from build123d import *

# Parameters (mm, degrees)
F0_W          = 140
F0_H          = 45
F1_DEPTH      = 20
F2_W          = 100
F2_H          = 27
F3_DEPTH      = 25
F4_R          = 2.65
F5_DEPTH      = 45.001
F6_R          = 4.5
F7_DEPTH      = 25
F8_T1_DEPTH   = 80
F9_R          = 5
F10_T1_DEPTH  = 116
F10_T3_DEPTH  = 90
F10_T5_DEPTH  = 37
F10_T7_DEPTH  = 48
F10_T10_ANGLE = 90
F10_T12_ANGLE = 90
F10_T14_ANGLE = 89.9999999987
F10_T16_ANGLE = 89.9999999987
F10_T18_ANGLE = 90
F10_T20_ANGLE = 90
F10_T22_ANGLE = 89.9999999987
F10_T24_ANGLE = 89.9999999987


# Not quite as in the source:
# - a fillet or chamfer that OpenCascade refuses, or shapes differently, is made with other operations: its cross-section is extruded or revolved along the edge and cut away or added


with BuildPart() as f1:
    # F0 (on Top) → F1 (new body)
    with BuildSketch(Plane.XY):
        Rectangle(F0_W, F0_H)
    extrude(amount=F1_DEPTH)

    # F2 (on face) → F3 (cut)
    with BuildSketch(Plane.XY.offset(20)):
        with Locations((0, -9)):
            Rectangle(F2_W, F2_H)
    extrude(amount=-F3_DEPTH, mode=Mode.SUBTRACT)

    # F4 (on face) → F5 (cut, through all)
    with BuildSketch(Plane(origin=(0, 22.5, 0), x_dir=(-1, 0, 0), z_dir=(0, 1, 0))):
        with Locations((60, 10)):
            Circle(F4_R)
        with Locations((-60, 10)):
            Circle(F4_R)
    extrude(amount=-F5_DEPTH, mode=Mode.SUBTRACT)

    # F6 (on face) → F7 (cut)
    with BuildSketch(Plane(origin=(0, 22.5, 0), x_dir=(-1, 0, 0), z_dir=(0, 1, 0))):
        with Locations((60, 10)):
            Circle(F6_R)
        with Locations((-60, 10)):
            Circle(F6_R)
    extrude(amount=-F7_DEPTH, mode=Mode.SUBTRACT)

    # F8: fillet of radius 12 on 2 edges, made by hand

    # F8_s2 → F8_t1 (cut)
    with BuildSketch(Plane.XY.offset(-30)):
        with BuildLine():
            ThreePointArc((-58, 22.5), (-66.4852813742, 18.9852813742), (-70, 10.5))
            Line((-70, 10.5), (-70, 22.5))
            Line((-70, 22.5), (-58, 22.5))
        make_face()
        with BuildLine():
            ThreePointArc((58, 22.5), (66.4852813742, 18.9852813742), (70, 10.5))
            Line((70, 10.5), (70, 22.5))
            Line((70, 22.5), (58, 22.5))
        make_face()
    extrude(amount=F8_T1_DEPTH, mode=Mode.SUBTRACT)

    # F9
    f9_edges = [f1.edges().sort_by_distance(p)[0] for p in [
        (-50, 4.5, 10),
        (50, 4.5, 10),
    ]]
    fillet(f9_edges, radius=F9_R)

    # F10: fillet of radius 6 on 20 edges, made by hand

    # F10_s2 → F10_t1 (cut)
    with BuildSketch(Plane.YZ.offset(-58)):
        with BuildLine():
            ThreePointArc((22.5, 14), (20.7426406871, 18.2426406871), (16.5, 20))
            Line((16.5, 20), (22.5, 20))
            Line((22.5, 20), (22.5, 14))
        make_face()
        with BuildLine():
            ThreePointArc((16.5, 0), (20.7426406871, 1.7573593129), (22.5, 6))
            Line((22.5, 6), (22.5, 0))
            Line((22.5, 0), (16.5, 0))
        make_face()
    extrude(amount=F10_T1_DEPTH, mode=Mode.SUBTRACT)

    # F10_s4 → F10_t3 (cut)
    with BuildSketch(Plane.YZ.offset(-45)):
        with BuildLine():
            ThreePointArc((4.5, 14), (6.2573593129, 18.2426406871), (10.5, 20))
            Line((10.5, 20), (4.5, 20))
            Line((4.5, 20), (4.5, 14))
        make_face()
        with BuildLine():
            ThreePointArc((10.5, 0), (6.2573593129, 1.7573593129), (4.5, 6))
            Line((4.5, 6), (4.5, 0))
            Line((4.5, 0), (10.5, 0))
        make_face()
    extrude(amount=F10_T3_DEPTH, mode=Mode.SUBTRACT)

    # F10_s6 → F10_t5 (cut)
    with BuildSketch(Plane.XZ.offset(0.5)):
        with BuildLine():
            ThreePointArc((56, 0), (51.7573593129, 1.7573593129), (50, 6))
            Line((50, 6), (50, 0))
            Line((50, 0), (56, 0))
        make_face()
        with BuildLine():
            ThreePointArc((-56, 0), (-51.7573593129, 1.7573593129), (-50, 6))
            Line((-50, 6), (-50, 0))
            Line((-50, 0), (-56, 0))
        make_face()
        with BuildLine():
            ThreePointArc((50, 14), (51.7573593129, 18.2426406871), (56, 20))
            Line((56, 20), (50, 20))
            Line((50, 20), (50, 14))
        make_face()
        with BuildLine():
            ThreePointArc((-50, 14), (-51.7573593129, 18.2426406871), (-56, 20))
            Line((-56, 20), (-50, 20))
            Line((-50, 20), (-50, 14))
        make_face()
    extrude(amount=F10_T5_DEPTH, mode=Mode.SUBTRACT)

    # F10_s8 → F10_t7 (cut)
    with BuildSketch(Plane.XZ.offset(-10.5)):
        with BuildLine():
            ThreePointArc((64, 0), (68.2426406871, 1.7573593129), (70, 6))
            Line((70, 6), (70, 0))
            Line((70, 0), (64, 0))
        make_face()
        with BuildLine():
            ThreePointArc((-64, 0), (-68.2426406871, 1.7573593129), (-70, 6))
            Line((-70, 6), (-70, 0))
            Line((-70, 0), (-64, 0))
        make_face()
        with BuildLine():
            ThreePointArc((70, 14), (68.2426406871, 18.2426406871), (64, 20))
            Line((64, 20), (70, 20))
            Line((70, 20), (70, 14))
        make_face()
        with BuildLine():
            ThreePointArc((-70, 14), (-68.2426406871, 18.2426406871), (-64, 20))
            Line((-64, 20), (-70, 20))
            Line((-70, 20), (-70, 14))
        make_face()
    extrude(amount=F10_T7_DEPTH, mode=Mode.SUBTRACT)

    # F10_s9 → F10_t10 (revolve, cut)
    with BuildSketch(Plane.XZ.offset(0.5)):
        with BuildLine():
            ThreePointArc((56, 0), (51.7573593129, 1.7573593129), (50, 6))
            Line((50, 6), (50, 0))
            Line((50, 0), (56, 0))
        make_face()
    revolve(axis=Axis((45, -0.5, 0), (0, 0, 1)), revolution_arc=F10_T10_ANGLE, mode=Mode.SUBTRACT)

    # F10_s11 → F10_t12 (revolve, cut)
    with BuildSketch(Plane.YZ.offset(-45)):
        with BuildLine():
            ThreePointArc((10.5, 0), (6.2573593129, 1.7573593129), (4.5, 6))
            Line((4.5, 6), (4.5, 0))
            Line((4.5, 0), (10.5, 0))
        make_face()
    revolve(axis=Axis((-45, -0.5, 0), (0, 0, 1)), revolution_arc=F10_T12_ANGLE, mode=Mode.SUBTRACT)

    # F10_s13 → F10_t14 (revolve, cut)
    with BuildSketch(Plane.YZ.offset(57.9999999999)):
        with BuildLine():
            ThreePointArc((16.5, 0), (20.7426406871, 1.7573593129), (22.5, 6))
            Line((22.5, 6), (22.5, 0))
            Line((22.5, 0), (16.5, 0))
        make_face()
    revolve(axis=Axis((57.9999999999, 10.4999999999, 0), (0, 0, -1)), revolution_arc=F10_T14_ANGLE, mode=Mode.SUBTRACT)

    # F10_s15 → F10_t16 (revolve, cut)
    with BuildSketch(Plane.XZ.offset(-10.4999999999)):
        with BuildLine():
            ThreePointArc((-64, 0), (-68.2426406871, 1.7573593129), (-70, 6))
            Line((-70, 6), (-70, 0))
            Line((-70, 0), (-64, 0))
        make_face()
    revolve(axis=Axis((-57.9999999999, 10.4999999999, 0), (0, 0, -1)), revolution_arc=F10_T16_ANGLE, mode=Mode.SUBTRACT)

    # F10_s17 → F10_t18 (revolve, cut)
    with BuildSketch(Plane.XZ.offset(0.5)):
        with BuildLine():
            ThreePointArc((50, 14), (51.7573593129, 18.2426406871), (56, 20))
            Line((56, 20), (50, 20))
            Line((50, 20), (50, 14))
        make_face()
    revolve(axis=Axis((45, -0.5, 20), (0, 0, 1)), revolution_arc=F10_T18_ANGLE, mode=Mode.SUBTRACT)

    # F10_s19 → F10_t20 (revolve, cut)
    with BuildSketch(Plane.YZ.offset(-45)):
        with BuildLine():
            ThreePointArc((4.5, 14), (6.2573593129, 18.2426406871), (10.5, 20))
            Line((10.5, 20), (4.5, 20))
            Line((4.5, 20), (4.5, 14))
        make_face()
    revolve(axis=Axis((-45, -0.5, 20), (0, 0, 1)), revolution_arc=F10_T20_ANGLE, mode=Mode.SUBTRACT)

    # F10_s21 → F10_t22 (revolve, cut)
    with BuildSketch(Plane.YZ.offset(57.9999999999)):
        with BuildLine():
            ThreePointArc((22.5, 14), (20.7426406871, 18.2426406871), (16.5, 20))
            Line((16.5, 20), (22.5, 20))
            Line((22.5, 20), (22.5, 14))
        make_face()
    revolve(axis=Axis((57.9999999999, 10.4999999999, 20), (0, 0, -1)), revolution_arc=F10_T22_ANGLE, mode=Mode.SUBTRACT)

    # F10_s23 → F10_t24 (revolve, cut)
    with BuildSketch(Plane.XZ.offset(-10.4999999999)):
        with BuildLine():
            ThreePointArc((-70, 14), (-68.2426406871, 18.2426406871), (-64, 20))
            Line((-64, 20), (-70, 20))
            Line((-70, 20), (-70, 14))
        make_face()
    revolve(axis=Axis((-57.9999999999, 10.4999999999, 20), (0, 0, -1)), revolution_arc=F10_T24_ANGLE, mode=Mode.SUBTRACT)


solid = f1.part
Can you work these out from the model? Positions are in its coordinate system, mm. A direction names the side the tool comes from. Give positions to 0.01 mm unless a question says otherwise; leave off trailing zeros. Order: outer loops, then holes, each group sorted by start corner. A loop starts at its lowest first (then second) coordinate and runs counter-clockwise, first axis right, second up. Notation, with made-up numbers: M -33,-5.75 L 3,-5.75 A16 cw 3,14.25 Z; hole C 20,-7 d10. An arc over 180 degrees is marked long. Use one line per item in the form item = value.
Item 1: If I drill on line 1 along X through (y, z) = (8.75, 10); line 2 along X through (y, z) = (-19, 9.75); line 3 along Z through (x, y) = (-60, -9), over which ranges is the centre line in solid material (lowest first)? Write a range as [from, to].
Values follow:
line_1 = [-70, -64.5], [-55.5, 55.5], [64.5, 70]
line_2 = [-70, -62.64], [-57.36, -50], [50, 57.36], [62.64, 70]
line_3 = [0, 7.35], [12.65, 20]
Item 2: If we section it at D-D, the plane y = 8.5: Count the separate pieces of the cut face and the enclosed holes in it, and give its area (3 significant figures).
Values follow:
separate_pieces = 1
enclosed_holes = 2
area = 2,580 mm^2
Item 3: If we section it at B-B, the plane z = 10: Write out the boundary of the cut face in (x, y), and give its area (3 significant figures).
Values follow:
outline = M -70,-22.5 L -62.65,-22.5 L -62.65,-2.5 L -64.5,-2.5 L -64.5,20.59 A12 ccw -70,10.5 Z; M -57.35,-22.5 L -50,-22.5 L -50,-0.5 A5 cw -45,4.5 L 45,4.5 A5 cw 50,-0.5 L 50,-22.5 L 57.35,-22.5 L 57.35,-2.5 L 55.5,-2.5 L 55.5,22.5 L -55.5,22.5 L -55.5,-2.5 L -57.35,-2.5 Z; M 62.65,-22.5 L 70,-22.5 L 70,10.5 A12 ccw 64.5,20.59 L 64.5,-2.5 L 62.65,-2.5 Z
area = 2,890 mm^2
Item 4: For faces 5 (the cylindrical face through (-48.5, 3.07, 9.94)), 6 (the cylindrical face through (51.804, -11.346, 1.711)), 7 (the cylindrical face through (-51.711, -11.346, 18.196)), 8 (the flat face through (-62, -2.5, 8)), which set-ups out of +Z, -Z, +X, -X, +Y, -Y let a thin tool reach every point of the face, with its end or its side?
Values follow:
face_5 = +Z, -Z, -Y
face_6 = -Z, -Y
face_7 = +Z, -Y
face_8 = +Y
Item 5: Thinking about a two-plate mould opening in X: for faces 1 (the cylindrical face through (-68.289, -5.769, 18.196)), 2 (the cylindrical face through (68.196, -5.769, 1.711)), 3 (the cylindrical face through (48.57, 3, 9.94)), 4 (the flat face through (-58, -22.5, 8)), which applies, pulls with the +X half, pulls with the -X half, needs draft (parallel to the pull), parting line crosses it, or undercut?
Values follow:
face_1 = pulls with the -X half
face_2 = pulls with the +X half
face_3 = undercut
face_4 = needs draft
Item 6: Will these pins go through, and if not, where does the flat tip stop? pin 1 Ø8 at (x, z) = (22.5, 11.5) entering from -Y; pin 2 Ø10 at (x, z) = (-58.5, 9) entering from +Y; pin 3 Ø5.5 at (x, z) = (60, 10) entering from +Y; pin 4 Ø1 at (x, z) = (43, 4.5) entering from +Y.
Values follow:
pin_1 = 4.5
pin_2 = 22.5
pin_3 = -2.5
pin_4 = 22.42
Item 7: If we section it at C-C, the plane x = -36: Write out the boundary of the cut face in (y, z), and give its area (3 significant figures).
Values follow:
outline = M 4.5,6 A6 ccw 10.5,0 L 16.5,0 A6 ccw 22.5,6 L 22.5,14 A6 ccw 16.5,20 L 10.5,20 A6 ccw 4.5,14 Z
area = 329 mm^2
Item 8: If we section it at A-A, the plane y = -9: Write out the boundary of the cut face in (x, z).
Values follow:
outline = M -70,6 A6 ccw -64,0 L -56,0 A6 ccw -50,6 L -50,14 A6 ccw -56,20 L -64,20 A6 ccw -70,14 Z; M 50,6 A6 ccw 56,0 L 64,0 A6 ccw 70,6 L 70,14 A6 ccw 64,20 L 56,20 A6 ccw 50,14 Z; hole C -60,10 d5.3; hole C 60,10 d5.3
